Build history of the part. All positions in model axes, mm. Round coordinates to 2 decimals unless told otherwise and drop trailing zeros. Order: outer loops, then holes, each group sorted by start corner. A loop starts at its lowest first (then second) coordinate and runs counter-clockwise, first axis right, second up. Notation, with made-up numbers: (86, 30) -> (101, 30) arc R23 cw to (101, 66) -> close; hole circle Ø7 at (-15, -12.5). An arc over 180 degrees is marked (long way). Answer as a JSON object with one key per item and string values.
Autodesk Inventor part; units mm, degrees
ref_plane "YZ Plane" through (0, 0, 0) normal (1, 0, 0) x (0, 1, 0)
ref_plane "XZ Plane" through (0, 0, 0) normal (0, 1, 0) x (-1, 0, 0)
ref_plane "XY Plane" through (0, 0, 0) normal (0, 0, 1) x (1, 0, 0)
sketch "Esboço1" plane through (0, 0, 0) normal (0, 0, 1) x (1, 0, 0)
  arc A0 (0, 12.7) -> (-12.7, 0) centre (0, 0) ccw
  circle A1 centre (-47.371, 39.2) radius 5.08
  line L0 (0, 0) -> (0, 58.6538)
  arc A2 (12.7, 0) -> (0, 12.7) centre (0, 0) ccw
  circle A3 centre (47.371, 39.2) radius 5.08
  line L1 (12.7, 0) -> (43.538, 2.698)
  line L2 (12.7, 0) -> (62.7, 0) construction
  arc A4 (60.071, 39.2) -> (34.671, 39.2) centre (47.371, 39.2) ccw
  line L3 (-12.7, 0) -> (-43.538, 2.698)
  arc A5 (-34.671, 39.2) -> (-60.071, 39.2) centre (-47.371, 39.2) ccw
  line L4 (34.671, 39.2) -> (34.671, 26.5)
  line L5 (-34.671, 39.2) -> (-34.671, 26.5)
  line L6 (60.071, 39.2) -> (60.071, 26.5)
  arc A6 (43.538, 2.698) -> (60.071, 26.5) centre (34.671, 26.5) ccw
  line L7 (-60.071, 39.2) -> (-60.071, 26.5)
  arc A7 (-60.071, 26.5) -> (-43.538, 2.698) centre (-34.671, 26.5) ccw
  line L8 (34.671, 26.5) -> (4.7852, 23.8853)
  line L9 (-34.671, 26.5) -> (-4.7852, 23.8853)
  arc A8 (-4.7852, 23.8853) -> (4.7852, 23.8853) centre (0, 74.0401) ccw
  point P0 (0, 25.2951)
  point P1 (0, 24.8739)
  dimension "d6" = 12.7
  dimension "d10" = 25.4
  dimension "d17" = 5
  dimension "d18" = 12.7
  dimension "d19" = 25.4
  dimension "d20" = 12.7
  dimension "d27" = 12.7
  dimension "d36" = 25.4
  dimension "d37" = 30
extrude "Extrusion2" add sketch "Esboço1" along normal blind 1.5
properties part number "FixaçãoTanque_1" material "Liga de aço"
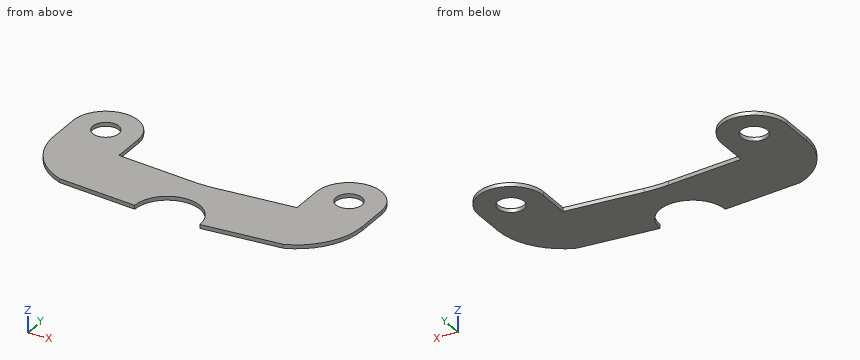
1) Flat gauge pins, fed straight in: pin 1 Ø9 at (x, y) = (47.371, 39.2) entering from +Z; pin 2 Ø6 at (x, y) = (-42, 41.5) entering from -Z. Where does each tip first touch, or does it go through?
Checked values:
{"pin 1": "passes through", "pin 2": "stops at z = 0"}
2) Probe L1, parallel to X at y = 29.5, z = 0.75; L2, parallel to Y at x = 44, z = 0.9; L3, parallel to X at y = 45.5, z = 1.25. List the from-to ranges inside material, lowest first. Write a range as from..to.
Checked values:
{"L1": "x = -60.07..-34.67, 34.67..60.07", "L2": "y = 2.88..35.4, 43..51.44", "L3": "x = -58.4..-36.34, 36.34..58.4"}
3) Cut at A-A, the plane y = 32.5. Give the cut face in (x, z), plus the area to 3 significant figures.
Checked values:
{"outline": "(-60.07, 0) -> (-34.67, 0) -> (-34.67, 1.5) -> (-60.07, 1.5) -> close; (34.67, 0) -> (60.07, 0) -> (60.07, 1.5) -> (34.67, 1.5) -> close", "area": "76.2 mm²"}
4) Cut at D-D, the plane x = 0. Give the cut face in (y, z).
Checked values:
{"outline": "(12.7, 0) -> (23.66, 0) -> (23.66, 1.5) -> (12.7, 1.5) -> close"}
5) Cut at B-B, the plane z = 0.9. Give the cut face in (x, y), plus the area to 3 significant figures.
Checked values:
{"outline": "(-60.07, 26.5) arc R25.4 ccw to (-43.54, 2.7) -> (-12.7, 0) arc R12.7 cw to (12.7, 0) -> (43.54, 2.7) arc R25.4 ccw to (60.07, 26.5) -> (60.07, 39.2) arc R12.7 ccw to (34.67, 39.2) -> (34.67, 26.5) -> (4.79, 23.89) arc R50.38 cw to (-4.79, 23.89) -> (-34.67, 26.5) -> (-34.67, 39.2) arc R12.7 ccw to (-60.07, 39.2) -> close; hole circle Ø10.16 at (-47.37, 39.2); hole circle Ø10.16 at (47.37, 39.2)", "area": "3,430 mm²"}
6) Cut at C-C, the plane x = -45. Give the cut face in (y, z), plus the area to 3 significant figures.
Checked values:
{"outline": "(3.3, 0) -> (34.71, 0) -> (34.71, 1.5) -> (3.3, 1.5) -> close; (43.69, 0) -> (51.68, 0) -> (51.68, 1.5) -> (43.69, 1.5) -> close", "area": "59.1 mm²"}
